```python
from build123d import *

# Parameters (mm, degrees)
RIGHTM_DEPTH = 30
LEFTM_START  = -30
LEFTM_DEPTH  = 30


with BuildPart() as part:
    # Sketch1 → rightM (new body)
    with BuildSketch(Plane.XY):
        Polygon((149.855864514, 43.874842), (149.855864514, 28.52351163), (192.119809278, 28.52351163), (234.383754043, 28.52351163), (234.383754043, 43.874842), (192.853964769, 43.874842), align=None)
        with BuildLine():
            Line((149.855864514, 28.52351163), (149.855864514, -58.067716007))
            ThreePointArc((149.855864514, -58.067716007), (156.250771623, -25.404082318), (174.491218383, 2.436426025))
            ThreePointArc((174.491218383, 2.436426025), (182.853494659, 9.95749243), (192.119809278, 16.331621214))
            Line((192.119809278, 16.331621214), (192.119809278, 28.52351163))
            Line((192.119809278, 28.52351163), (149.855864514, 28.52351163))
        make_face()
        with BuildLine():
            Line((107.405043491, 43.874842), (94.874715104, -28.778692489))
            add(Edge.make_bspline(
                [(94.874715104, -28.778692489), (125.81929731, -36.765852729), (149.855864514, -58.067716007)],
                knots=[0, 0, 0, 1, 1, 1], degree=2))
            Line((149.855864514, -58.067716007), (149.855864514, 43.874842))
            Line((149.855864514, 43.874842), (107.405043491, 43.874842))
        make_face()
    extrude(amount=RIGHTM_DEPTH)

    # Sketch2 → leftM (add)
    with BuildSketch(Plane.XY.offset(LEFTM_START)):
        Polygon((149.855864514, 43.874842), (149.855864514, 28.52351163), (192.119809278, 28.52351163), (234.383754043, 28.52351163), (234.383754043, 43.874842), (192.853964769, 43.874842), align=None)
        with BuildLine():
            Line((107.405043491, 43.874842), (94.874715104, -28.778692489))
            add(Edge.make_bspline(
                [(94.874715104, -28.778692489), (125.81929731, -36.765852729), (149.855864514, -58.067716007)],
                knots=[0, 0, 0, 1, 1, 1], degree=2))
            Line((149.855864514, -58.067716007), (149.855864514, 43.874842))
            Line((149.855864514, 43.874842), (107.405043491, 43.874842))
        make_face()
        with BuildLine():
            Line((149.855864514, 28.52351163), (149.855864514, -58.067716007))
            ThreePointArc((149.855864514, -58.067716007), (156.250771623, -25.404082318), (174.491218383, 2.436426025))
            ThreePointArc((174.491218383, 2.436426025), (182.853494659, 9.95749243), (192.119809278, 16.331621214))
            Line((192.119809278, 16.331621214), (192.119809278, 28.52351163))
            Line((192.119809278, 28.52351163), (149.855864514, 28.52351163))
        make_face()
    extrude(amount=LEFTM_DEPTH)


solid = part.part
```
Build history of the part. All positions in model axes, mm. A direction names the side the tool comes from. Give positions to 0.01 mm unless a question says otherwise; leave off trailing zeros. Order: outer loops, then holes, each group sorted by start corner. A loop starts at its lowest first (then second) coordinate and runs counter-clockwise, first axis right, second up. Notation, with made-up numbers: M 66,-40 L 76,-40 A7 ccw 76,-33 Z; hole C 22,14.25 d3. An arc over 180 degrees is marked long. Return JSON: item names as keys, results as strings.
Q1. 3-axis set-ups, long thin cutter, end or side, ignore diameter. For faces 1 (the face through (213, 28.524, 0)), 2 (the face through (172, 43.875, 0)): which of +Z, -Z, +X, -X, +Y, -Y reach the whole face in a straight line?
Answer list:
{"face 1": "+Z, -Z, +X, -Y", "face 2": "+Z, -Z, +X, -X, +Y"}
Q2. Band-saw the part on B-B (y = -4.5). Give the cut face in (x, z), then the cut area to 3 significant figures.
Answer list:
{"outline": "M 99.06,-30 L 168.41,-30 L 168.41,30 L 99.06,30 Z", "area": "4,160 mm^2"}
Q3. Wall check: probe 1 along Y at (x, z) = (207.5, -20); probe 2 along X at (y, z) = (-43.5, 3); probe 3 along X at (y, z) = (-16, -4). Give the ranges that are in metal, low to high. Write a range as from..to.
Answer list:
{"probe 1": "y = 28.52..43.87", "probe 2": "x = 130.09..151.09", "probe 3": "x = 97.08..160.76"}
Q4. Flat gauge pins, fed straight in: pin 1 (10 mm diameter, centred on y = -41.5, z = 23, fed in from -X); pin 2 (12.5 mm diameter, centred on x = 208, z = 5.5, fed in from -Y); pin 3 (1.5 mm diameter, centred on x = 175, z = -13.5, fed in from -Y); pin 4 (10 mm diameter, centred on x = 164, y = -13, fed in from +Z). Where does each tip first touch, or does it go through?
Answer list:
{"pin 1": "stops at x = 116.8", "pin 2": "stops at y = 28.52", "pin 3": "stops at y = 2.19", "pin 4": "stops at z = 30"}
Q5. Band-saw the part on A-A (x = 210). Give the cut face in (y, z).
Answer list:
{"outline": "M 28.52,-30 L 43.87,-30 L 43.87,30 L 28.52,30 Z"}
